from build123d import *

# Parameters (mm, degrees)
SKETCH_1_R          = 1
EXTRUDE_1_DEPTH     = 3.8
SKETCH_2_W          = 13
SKETCH_2_H          = 10
CUT_EXTRUDE_1_DEPTH = 3.3


with BuildPart() as part:
    # Эскиз1 → Бобышка-Вытянуть1 (new body)
    with BuildSketch(Plane.XY):
        with BuildLine():
            Line((-9.75, 5), (11.75, 5))
            Line((11.75, 5), (11.75, -5))
            Line((11.75, -5), (-9.75, -5))
            ThreePointArc((-9.75, -5), (-11.164213562, -4.414213562), (-11.75, -3))
            Line((-11.75, -3), (-11.75, 3))
            ThreePointArc((-11.75, 3), (-11.164213562, 4.414213562), (-9.75, 5))
        make_face()
        with Locations((-9.538461538, 0)):
            Circle(SKETCH_1_R, mode=Mode.SUBTRACT)
    extrude(amount=EXTRUDE_1_DEPTH)

    # Эскиз2 → Вырез-Вытянуть1 (cut)
    with BuildSketch(Plane.XY.offset(3.8)):
        with Locations((5.25, 0)):
            Rectangle(SKETCH_2_W, SKETCH_2_H)
    extrude(amount=-CUT_EXTRUDE_1_DEPTH, mode=Mode.SUBTRACT)


solid = part.part
Read the model definition and answer for the solid it produces. Units are mm, in the model's axes. A direction names the side the tool comes from. Round coordinates to 2 decimals unless told otherwise and drop trailing zeros. Order: outer loops, then holes, each group sorted by start corner. A loop starts at its lowest first (then second) coordinate and runs counter-clockwise, first axis right, second up.
1) The part is cut by section D-D on y = 4.25. Write down the section's boundary in (x, z), plus the area to 3 significant figures.
2) Straight lines are drawn through the part: L1, parallel to X at y = -3, z = 1.65; L2, parallel to Z at x = 1.25, y = 2; L3, parallel to Y at x = -10, z = 1.15. For each, find the intervals that lie inside material, in ascending order.
3) The part is cut by section A-A on y = 0. Write down the section's boundary in (x, z), plus the area to 3 significant figures.
4) The mould has two halves that part along X. Classify faces 1 (the face through (-4, 5, 2)), 2 (the face through (-11.18, 4.4, 1.87)), 3 (the face through (-8.585, 0.3, 1.873)): released by +X, released by -X, zero draft, split by the parting line, or undercut.
5) The part is cut by section C-C on x = 3.25. Write down the section's boundary in (y, z), plus the area to 3 significant figures.
6) For faces 4 (the face through (-11.15, -4.43, 1.87)), 5 (the face through (-1.25, 0, 2)), determine the directions among +Z, -Z, +X, -X, +Y, -Y from which every point of the face is accessible in a straight line to the end or side of a thin tool.
7) The part is cut by section B-B on z = 1.55. Write down the section's boundary in (x, y), plus the area to 3 significant figures.
8) Flat-ended cylindrical pins translate along their axes: pin 1 (1 mm diameter, centred on y = 2, z = 2, fed in from +X); pin 2 (6 mm diameter, centred on x = 2, y = 1, fed in from -Z); pin 3 (6 mm diameter, centred on x = 6.5, y = -2.5, fed in from +Z). Find the tip coordinate at first contact, or state that the pin passes through.
Resolved:
1. outline: (-11.31, 0) - (11.75, 0) - (11.75, 0.5) - (-1.25, 0.5) - (-1.25, 3.8) - (-11.31, 3.8) - close
1. area: 44.7 mm2
2. L1: x = -11.75 to -1.25
2. L2: z = 0 to 0.5
2. L3: y = -4.98 to -0.89, 0.89 to 4.98
3. outline: (-11.75, 0) - (-10.54, 0) - (-10.54, 3.8) - (-11.75, 3.8) - close; (-8.54, 0) - (11.75, 0) - (11.75, 0.5) - (-1.25, 0.5) - (-1.25, 3.8) - (-8.54, 3.8) - close
3. area: 38.8 mm2
4. face 1: zero draft
4. face 2: released by -X
4. face 3: undercut
5. outline: (-5, 0) - (5, 0) - (5, 0.5) - (-5, 0.5) - close
5. area: 5.00 mm2
6. face 4: +Z, -Z, -X, -Y
6. face 5: +Z, +X, +Y, -Y
7. outline: (-11.75, -3) arc R2 ccw to (-9.75, -5) - (-1.25, -5) - (-1.25, 5) - (-9.75, 5) arc R2 ccw to (-11.75, 3) - close; hole circle Ø2 at (-9.54, 0)
7. area: 100 mm2
8. pin 1: stops at x = -1.25
8. pin 2: stops at z = 0
8. pin 3: stops at z = 0.5
